from build123d import *

# Parameters (mm, degrees)
SKETCH2_W           = 41.275
SKETCH2_H           = 29.464
BOSS_EXTRUDE1_DEPTH = 8.89
BOSS_EXTRUDE2_DEPTH = 29.14396
SKETCH6_R           = 1.5
CUT_EXTRUDE1_DEPTH  = 6.5
SKETCH7_R           = 1.5
CUT_EXTRUDE2_DEPTH  = 6
SKETCH8_R           = 1.885
SKETCH8_R_2         = 1.25
EXTRUDE_THIN1_DEPTH = 2
CUT_EXTRUDE3_START  = -21.78
SKETCH8_3_R         = 1.25
CUT_EXTRUDE3_DEPTH  = 21.78
CUT_EXTRUDE4_START  = -82.9
SKETCH7_2_R         = 1.5
CUT_EXTRUDE4_DEPTH  = 6
SKETCH9_W           = 12.7
SKETCH9_H           = 16.51
CUT_EXTRUDE5_DEPTH  = 6.35
CUT_EXTRUDE6_START  = -177.8
SKETCH9_2_W         = 12.7
SKETCH9_2_H         = 16.51
CUT_EXTRUDE6_DEPTH  = 6.35
SKETCH10_R          = 1
CUT_EXTRUDE8_DEPTH  = 2


with BuildPart() as part:
    # Sketch2 → Boss-Extrude1 (new body)
    with BuildSketch(Plane(origin=(0, 0, 0), x_dir=(1, 0, 0), z_dir=(0, 1, 0))):
        with Locations((26.9875, 74.168)):
            Rectangle(SKETCH2_W, SKETCH2_H)
        with Locations((26.9875, 14.732)):
            Rectangle(SKETCH2_W, SKETCH2_H)
        Polygon((0, 88.9), (0, 0), (6.35, 0), (6.35, 29.464), (47.625, 29.464), (47.625, 0), (53.975, 0), (53.975, 12.7), (53.975, 76.2), (53.975, 88.9), (47.625, 88.9), (47.625, 59.436), (6.35, 59.436), (6.35, 88.9), align=None)
        Polygon((53.975, 12.7), (69.85, 12.7), (107.95, 12.7), (123.825, 12.7), (123.825, 76.2), (107.95, 76.2), (69.85, 76.2), (53.975, 76.2), align=None)
        Polygon((53.975, 12.7), (53.975, 0), (69.85, 12.7), align=None)
        Polygon((107.95, 12.7), (123.825, 0), (123.825, 12.7), align=None)
        Polygon((123.825, 12.7), (123.825, 0), (130.175, 0), (130.175, 29.464), (171.45, 29.464), (171.45, 0), (177.8, 0), (177.8, 88.9), (171.45, 88.9), (171.45, 59.436), (130.175, 59.436), (130.175, 88.9), (123.825, 88.9), (123.825, 76.2), align=None)
        with Locations((150.8125, 14.732)):
            Rectangle(SKETCH2_W, SKETCH2_H)
        with Locations((150.8125, 74.168)):
            Rectangle(SKETCH2_W, SKETCH2_H)
        Polygon((123.825, 76.2), (123.825, 88.9), (107.95, 76.2), align=None)
        Polygon((69.85, 76.2), (53.975, 88.9), (53.975, 76.2), align=None)
    extrude(amount=BOSS_EXTRUDE1_DEPTH)

    # Sketch2<3> → Boss-Extrude2 (add)
    with BuildSketch(Plane(origin=(0, 0, 0), x_dir=(1, 0, 0), z_dir=(0, 1, 0))):
        Polygon((0, 88.9), (0, 0), (6.35, 0), (6.35, 29.464), (47.625, 29.464), (47.625, 0), (53.975, 0), (53.975, 12.7), (53.975, 76.2), (53.975, 88.9), (47.625, 88.9), (47.625, 59.436), (6.35, 59.436), (6.35, 88.9), align=None)
        Polygon((123.825, 12.7), (123.825, 0), (130.175, 0), (130.175, 29.464), (171.45, 29.464), (171.45, 0), (177.8, 0), (177.8, 88.9), (171.45, 88.9), (171.45, 59.436), (130.175, 59.436), (130.175, 88.9), (123.825, 88.9), (123.825, 76.2), align=None)
    extrude(amount=BOSS_EXTRUDE2_DEPTH)

    # Sketch6 → Cut-Extrude1 (cut)
    with BuildSketch(Plane(origin=(0, 29.14396, 0), x_dir=(1, 0, 0), z_dir=(0, 1, 0))):
        with Locations(Location((26.9875, 44.45, 0), (0, 0, 270))):
            Circle(SKETCH6_R)
        with Locations(Location((150.8125, 44.45, 0), (0, 0, 270))):
            Circle(SKETCH6_R)
    extrude(amount=-CUT_EXTRUDE1_DEPTH, mode=Mode.SUBTRACT)

    # Sketch7 → Cut-Extrude2 (cut)
    with BuildSketch(Plane.XY):
        with Locations((2.4375, 14.04)):
            Circle(SKETCH7_R)
        with Locations((51.5375, 14.04)):
            Circle(SKETCH7_R)
        with Locations((2.4375, 23.740006)):
            Circle(SKETCH7_R)
        with Locations((51.5375, 23.740006)):
            Circle(SKETCH7_R)
        with Locations(Location((126.2625, 23.740006, 0), (0, 0, 180))):
            Circle(SKETCH7_R)
        with Locations(Location((175.3625, 23.740006, 0), (0, 0, 180))):
            Circle(SKETCH7_R)
        with Locations(Location((126.2625, 14.04, 0), (0, 0, 180))):
            Circle(SKETCH7_R)
        with Locations(Location((175.3625, 14.04, 0), (0, 0, 180))):
            Circle(SKETCH7_R)
    extrude(amount=-CUT_EXTRUDE2_DEPTH, mode=Mode.SUBTRACT)

    # Sketch8 → Extrude-Thin1 (add)
    # profile 1 of 4: a face of its own
    with BuildSketch(Plane(origin=(0, 8.89, 0), x_dir=(1, 0, 0), z_dir=(0, 1, 0))):
        with Locations((61.087, 53.975)):
            Circle(SKETCH8_R)
        with Locations((61.087, 53.975)):
            Circle(SKETCH8_R_2, mode=Mode.SUBTRACT)
    # profile 2 of 4: a face of its own
    with BuildSketch(Plane(origin=(0, 8.89, 0), x_dir=(1, 0, 0), z_dir=(0, 1, 0))):
        with Locations((61.087, 34.925)):
            Circle(SKETCH8_R)
        with Locations((61.087, 34.925)):
            Circle(SKETCH8_R_2, mode=Mode.SUBTRACT)
    # profile 3 of 4: a face of its own
    with BuildSketch(Plane(origin=(0, 8.89, 0), x_dir=(1, 0, 0), z_dir=(0, 1, 0))):
        with Locations((116.713, 34.925)):
            Circle(SKETCH8_R)
        with Locations((116.713, 34.925)):
            Circle(SKETCH8_R_2, mode=Mode.SUBTRACT)
    # profile 4 of 4: a face of its own
    with BuildSketch(Plane(origin=(0, 8.89, 0), x_dir=(1, 0, 0), z_dir=(0, 1, 0))):
        with Locations((116.713, 53.975)):
            Circle(SKETCH8_R)
        with Locations((116.713, 53.975)):
            Circle(SKETCH8_R_2, mode=Mode.SUBTRACT)
    extrude(amount=EXTRUDE_THIN1_DEPTH)

    # Sketch8<3> → Cut-Extrude3 (cut)
    with BuildSketch(Plane(origin=(0, 8.89, 0), x_dir=(1, 0, 0), z_dir=(0, 1, 0)).offset(CUT_EXTRUDE3_START)):
        with Locations(Location((61.087, 53.975, 0), (0, 0, 270))):
            Circle(SKETCH8_3_R)
        with Locations(Location((61.087, 34.925, 0), (0, 0, 270))):
            Circle(SKETCH8_3_R)
        with Locations(Location((116.713, 34.925, 0), (0, 0, 270))):
            Circle(SKETCH8_3_R)
        with Locations(Location((116.713, 53.975, 0), (0, 0, 270))):
            Circle(SKETCH8_3_R)
    extrude(amount=CUT_EXTRUDE3_DEPTH, mode=Mode.SUBTRACT)

    # Sketch7<2> → Cut-Extrude4 (cut)
    with BuildSketch(Plane.XY.offset(CUT_EXTRUDE4_START)):
        with Locations((2.4375, 14.04)):
            Circle(SKETCH7_2_R)
        with Locations((51.5375, 14.04)):
            Circle(SKETCH7_2_R)
        with Locations((2.4375, 23.740006)):
            Circle(SKETCH7_2_R)
        with Locations((51.5375, 23.740006)):
            Circle(SKETCH7_2_R)
        with Locations(Location((126.2625, 23.740006, 0), (0, 0, 180))):
            Circle(SKETCH7_2_R)
        with Locations(Location((175.3625, 23.740006, 0), (0, 0, 180))):
            Circle(SKETCH7_2_R)
        with Locations(Location((126.2625, 14.04, 0), (0, 0, 180))):
            Circle(SKETCH7_2_R)
        with Locations(Location((175.3625, 14.04, 0), (0, 0, 180))):
            Circle(SKETCH7_2_R)
    extrude(amount=-CUT_EXTRUDE4_DEPTH, mode=Mode.SUBTRACT)

    # Sketch9 → Cut-Extrude5 (cut)
    with BuildSketch(Plane.ZY):
        with Locations((-23.114, 20.88896)):
            Rectangle(SKETCH9_W, SKETCH9_H)
        with Locations((-65.786, 20.88896)):
            Rectangle(SKETCH9_W, SKETCH9_H)
    extrude(amount=-CUT_EXTRUDE5_DEPTH, mode=Mode.SUBTRACT)

    # Sketch9<2> → Cut-Extrude6 (cut)
    with BuildSketch(Plane.ZY.offset(CUT_EXTRUDE6_START)):
        with Locations((-23.114, 20.88896)):
            Rectangle(SKETCH9_2_W, SKETCH9_2_H)
        with Locations((-65.786, 20.88896)):
            Rectangle(SKETCH9_2_W, SKETCH9_2_H)
    extrude(amount=CUT_EXTRUDE6_DEPTH, mode=Mode.SUBTRACT)

    # Sketch10 → Cut-Extrude8 (cut)
    with BuildSketch(Plane.ZY):
        with Locations((-54.991, 25.46096)):
            Circle(SKETCH10_R)
        with Locations((-33.909, 25.46096)):
            Circle(SKETCH10_R)
        with Locations((-33.909, 15.80896)):
            Circle(SKETCH10_R)
        with Locations((-54.991, 15.80896)):
            Circle(SKETCH10_R)
    extrude(amount=-CUT_EXTRUDE8_DEPTH, mode=Mode.SUBTRACT)


solid = part.part
Work out the finished part from the listing and answer in its coordinate system (mm). A direction names the side the tool comes from. Round coordinates to 2 decimals unless told otherwise and drop trailing zeros. Order: outer loops, then holes, each group sorted by start corner. A loop starts at its lowest first (then second) coordinate and runs counter-clockwise, first axis right, second up. Notation, with made-up numbers: M -30,-11.5 L 21,-11.5 A21 cw 21,-6.5 Z; hole C 52,58.5 d2. An arc over 180 degrees is marked long. Put each result on its own line as item: value. Start each with the question number.
Q1. Section C-C, the plane z = -67.5 is taken. Write down the section's boundary in (x, y) (3 decimals).
Q2. Straight lines are drawn through the part: L1, parallel to X at y = 20.25, z = -14 (3 decimals); L2, parallel to X at y = 26.25, z = -68.5 (3 decimals); L3, parallel to X at y = 20.75, z = -47 (3 decimals). For each, find the intervals that lie inside material, in ascending order. Write a range as [from, to].
Q3. Section D-D, the plane x = 75.5 is taken. Write down the section's boundary in (y, z).
Q4. A tool of negligible diameter and unlimited length cuts with its end or side. For faces 4 (the cylindrical face through (116.304, 9.876, -33.085)), 5 (the flat face through (115, 10.89, -35)), 6 (the flat face through (3, 21, -16.764)), from which of +Z, -Z, +X, -X, +Y, -Y can it reach the whole face along a straight path? Write none if from no direction.
Q5. For a pull along Z with two mould halves and no side action, classify faces 1 (the flat face through (27, 8, -88.9)), 2 (the flat face through (89, 4, -12.7)), 3 (the cylindrical face through (62.828, 9.876, -34.203)) as pulls with the +Z half, pulls with the -Z half, needs draft (parallel to the pull), parting line crosses it, or undercut.
Q6. Flat-ended cylindrical pins translate along their axes: pin 1 (10 mm diameter, centred on x = 80.5, y = 4.5, fed in from -Z); pin 2 (1.8 mm diameter, centred on x = 2.44, y = 23.74, fed in from +Z); pin 3 (3 mm diameter, centred on x = 61.087, z = -53.975, fed in from +Y). Find the tip coordinate at first contact, or state that the pin passes through.
Q7. Section B-B, the plane x = 11 is taken. Write down the section's boundary in (y, z), and give its area (3 significant figures).
Q8. Section A-A, the plane z = -81 is taken. Write down the section's boundary in (x, y) (3 decimals).
Findings below:
1. outline: M 0,0 L 177.8,0 L 177.8,12.634 L 171.45,12.634 L 171.45,8.89 L 130.175,8.89 L 130.175,29.144 L 123.825,29.144 L 123.825,8.89 L 53.975,8.89 L 53.975,29.144 L 47.625,29.144 L 47.625,8.89 L 6.35,8.89 L 6.35,12.634 L 0,12.634 Z
2. L1: x = [0, 6.35], [47.625, 53.975], [123.825, 130.175], [171.45, 177.8]
2. L2: x = [47.625, 53.975], [123.825, 130.175]
2. L3: x = [0, 53.975], [123.825, 177.8]
3. outline: M 0,-76.2 L 8.89,-76.2 L 8.89,-12.7 L 0,-12.7 Z
4. face 4: +Y
4. face 5: +Z, -Z, +Y
4. face 6: -X, +Y
5. face 1: pulls with the -Z half
5. face 2: pulls with the +Z half
5. face 3: undercut
6. pin 1: stops at z = -76.2
6. pin 2: stops at z = -6
6. pin 3: stops at y = 10.89
7. outline: M 0,-88.9 L 8.89,-88.9 L 8.89,-59.44 L 29.14,-59.44 L 29.14,-29.46 L 8.89,-29.46 L 8.89,0 L 0,0 Z
7. area: 1,400 mm^2
8. outline: M 0,0 L 63.85,0 L 63.85,8.89 L 53.975,8.89 L 53.975,29.144 L 47.625,29.144 L 47.625,8.89 L 6.35,8.89 L 6.35,29.144 L 0,29.144 Z; M 113.95,0 L 177.8,0 L 177.8,29.144 L 171.45,29.144 L 171.45,8.89 L 130.175,8.89 L 130.175,29.144 L 123.825,29.144 L 123.825,8.89 L 113.95,8.89 Z
